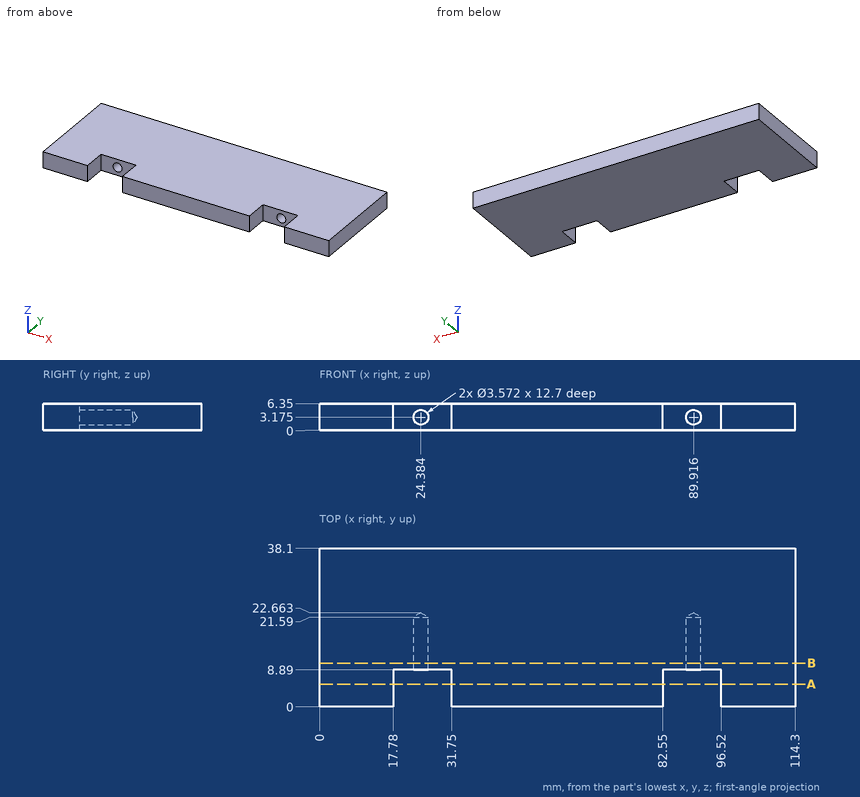
Print and shaded views of the part. All mm, measured from the part's lowest x, y and z. Round coordinates to 2 decimals unless told otherwise and drop trailing zeros. Loops run counter-clockwise (first coordinate to the right, second up) from the corner with the lowest first, then second, coordinate; pieces in that order, holes last. Notation, with made-up numbers: (7, -23) -> (22, -23) arc R27 ccw to (22, 5) -> close; hole circle Ø4 at (16, 26.5). An arc over 180 degrees is marked (long way). Use CSV: the item, a comma, the result in double quotes. Start each with the question number.
1) Cut at B-B, the plane y = 10.5. Write the cut outline in (x, z) (3 decimals).
2) Wall check: L1, parallel to X at y = 6, z = 6.25; L2, parallel to X at y = 21, z = 2; L3, parallel to Y at x = 30.5, z = 1.25. Give the ranges that are in metal, low to high. Write a range as [from, to].
3) Cut at A-A, the plane y = 5.5. Write the cut outline in (x, z), plus the area to 3 significant figures.
4) Drop flat-ended pins along their axis: P1, Ø3, axis at x = 91, z = 2.5, coming from the -Y side; P2, Ø3, axis at x = 24.384, z = 3.175, coming from the -Y side; P3, Ø2, axis at x = 89.916, z = 3.175, coming from the -Y side. Give the stop position or say it passes through.
Determined:
1,outline,"(0, 0) -> (114.3, 0) -> (114.3, 6.35) -> (0, 6.35) -> close; hole circle Ø3.572 at (24.384, 3.175); hole circle Ø3.572 at (89.916, 3.175)"
2,L1,"x = [0, 17.78], [31.75, 82.55], [96.52, 114.3]"
2,L2,"x = [0, 23.04], [25.73, 88.57], [91.26, 114.3]"
2,L3,"y = [8.89, 38.1]"
3,outline,"(0, 0) -> (17.78, 0) -> (17.78, 6.35) -> (0, 6.35) -> close; (31.75, 0) -> (82.55, 0) -> (82.55, 6.35) -> (31.75, 6.35) -> close; (96.52, 0) -> (114.3, 0) -> (114.3, 6.35) -> (96.52, 6.35) -> close"
3,area,"548 mm2"
4,P1,"stops at y = 8.89"
4,P2,"stops at y = 21.76"
4,P3,"stops at y = 22.06"
